from build123d import *

# Parameters (mm, degrees)
BOSS_EXTRUDE1_DEPTH = 3


with BuildPart() as part:
    # Model → Boss-Extrude1 (new body)
    with BuildSketch(Plane.XY):
        with BuildLine():
            Line((1159.8, -200.422661621), (1159.8, -247.652661621))
            Line((1159.8, -247.652661621), (1130.6, -247.652661621))
            Line((1130.6, -247.652661621), (1130.6, -227.655293314))
            ThreePointArc((1130.6, -227.655293314), (1099.799999997, -258.052661621), (1130.6, -288.450029928))
            Line((1130.6, -288.450029928), (1130.6, -268.452661621))
            Line((1130.6, -268.452661621), (1159.8, -268.452661621))
            Line((1159.8, -268.452661621), (1159.8, -315.682652611))
            add(Edge.make_bspline(
                [(1159.8, -315.682652611), (982.299469587, -317.054252859), (804.800894245, -318.714261239), (449.798296518, -321.162775901), (272.233603405, -323.726378565), (94.901037796, -315.441313757)],
                knots=[0, 0, 0, 0, 0.5, 0.5, 1, 1, 1, 1], degree=3))
            Line((94.901037796, -315.441313757), (94.901037796, -245.979700014))
            Line((94.901037796, -245.979700014), (97.901037796, -245.979700014))
            Line((97.901037796, -245.979700014), (97.901037796, -200.422661621))
            Line((97.901037796, -200.422661621), (253.901037796, -200.422661621))
            Line((253.901037796, -200.422661621), (253.901037796, -245.979700014))
            Line((253.901037796, -245.979700014), (256.901037795, -245.979700014))
            Line((256.901037795, -245.979700014), (256.901037795, -200.422661621))
            Line((256.901037795, -200.422661621), (412.901037795, -200.422661621))
            Line((412.901037795, -200.422661621), (412.901037795, -245.979700014))
            Line((412.901037795, -245.979700014), (415.901037795, -245.979700014))
            Line((415.901037795, -245.979700014), (415.901037795, -200.422661621))
            Line((415.901037795, -200.422661621), (571.901037795, -200.422661621))
            Line((571.901037795, -200.422661621), (571.901037795, -245.979700014))
            Line((571.901037795, -245.979700014), (574.901037795, -245.979700014))
            Line((574.901037795, -245.979700014), (574.901037795, -200.422661621))
            Line((574.901037795, -200.422661621), (730.901037795, -200.422661621))
            Line((730.901037795, -200.422661621), (730.901037795, -245.979700014))
            Line((730.901037795, -245.979700014), (733.901037795, -245.979700014))
            Line((733.901037795, -245.979700014), (733.901037795, -200.422661621))
            Line((733.901037795, -200.422661621), (889.901037795, -200.422661621))
            Line((889.901037795, -200.422661621), (889.901037795, -245.979700014))
            Line((889.901037795, -245.979700014), (892.901037795, -245.979700014))
            Line((892.901037795, -245.979700014), (892.901037795, -200.422661621))
            Line((892.901037795, -200.422661621), (1048.901037796, -200.422661621))
            Line((1048.901037796, -200.422661621), (1048.901037796, -245.979700014))
            Line((1048.901037796, -245.979700014), (1051.901037795, -245.979700014))
            Line((1051.901037795, -245.979700014), (1051.901037795, -200.422661621))
            Line((1051.901037795, -200.422661621), (1159.8, -200.422661621))
        make_face()
    extrude(amount=BOSS_EXTRUDE1_DEPTH)


solid = part.part
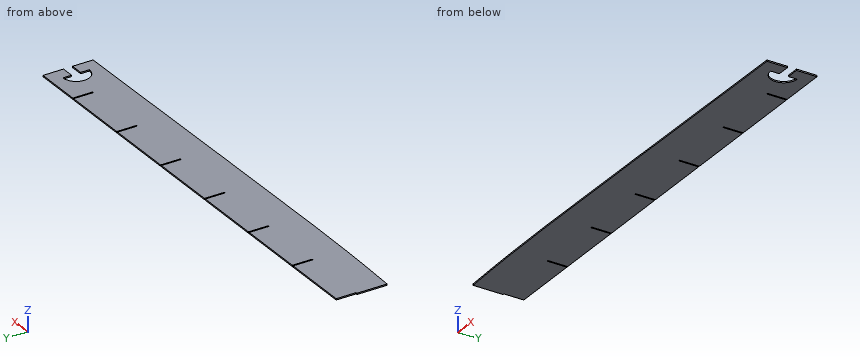
Here's how the part is built. I have some questions about the finished solid (model axes, mm). Coordinates: 2 decimals unless noted, no trailing zeros. Write each loop counter-clockwise with the first axis right and the second up, starting at its lowest first coordinate (ties: lowest second). Pieces come first, ordered by that corner, then holes. Notation, with made-up numbers: (-14, -7.5) - (20, -7.5) arc R23 cw to (20, 9.5) - close; hole circle Ø4 at (70, 28). An arc over 180 degrees is marked (long way). Use one line per item in the form item = value.
1) Suppose I cut it at A-A, the plane y = -210. Write out the boundary of the cut face in (x, z).
Solved:
outline = (97.9, 0) - (253.9, 0) - (253.9, 3) - (97.9, 3) - close; (256.9, 0) - (412.9, 0) - (412.9, 3) - (256.9, 3) - close; (415.9, 0) - (571.9, 0) - (571.9, 3) - (415.9, 3) - close; (574.9, 0) - (730.9, 0) - (730.9, 3) - (574.9, 3) - close; (733.9, 0) - (889.9, 0) - (889.9, 3) - (733.9, 3) - close; (892.9, 0) - (1048.9, 0) - (1048.9, 3) - (892.9, 3) - close; (1051.9, 0) - (1159.8, 0) - (1159.8, 3) - (1051.9, 3) - close
2) I'm going to push flat-ended pins straight in: P1, Ø1.5, axis at x = 608.5, y = -267, coming from the -Z side; P2, Ø1.5, axis at x = 256, z = 1.5, coming from the +Y side; P3, Ø0.9, axis at y = -217.5, z = 1.5, coming from the -X side. Where does each tip first touch, or does it pass through?
Solved:
P1 = 0
P2 = -245.98
P3 = 97.9
3) I need wall thicknesses on line 1 (X direction, y = -272, z = 1.2); line 2 (X direction, y = -256, z = 2.6); line 3 (Y direction, x = 337, z = 2.35). Which ranges of each line are inside material? Lowest first, please.
Solved:
line_1 = 94.9 to 1103.19, 1130.6 to 1159.8
line_2 = 94.9 to 1099.87
line_3 = -321.16 to -200.42
